from build123d import *

# Parameters (mm, degrees)
F0_R     = 10
F1_DEPTH = 25
F2_DEPTH = 50
F3_SIZE  = 2


with BuildPart() as f1:
    # F0 (on Front) → F1 (new body)
    with BuildSketch(Plane.XZ):
        with BuildLine():
            ThreePointArc((2.083333, -24.913043), (18.399502, -16.92508), (25, 0))
            ThreePointArc((25, 0), (18.399502, 16.92508), (2.083333, 24.913043))
            ThreePointArc((2.083333, 24.913043), (-25, 0), (2.083333, -24.913043))
        make_face()
        Circle(F0_R, mode=Mode.SUBTRACT)
        with BuildLine():
            ThreePointArc((2.083333, 24.913043), (18.399502, 16.92508), (25, 0))
            ThreePointArc((25, 0), (18.399502, -16.92508), (2.083333, -24.913043))
            Line((2.083333, -24.913043), (91.458333, -17.43913))
            ThreePointArc((91.458333, -17.43913), (72.5, 0), (91.458333, 17.43913))
            Line((91.458333, 17.43913), (2.083333, 24.913043))
        make_face()
        with BuildLine():
            ThreePointArc((107.5, 0), (102.879651, 11.847556), (91.458333, 17.43913))
            ThreePointArc((91.458333, 17.43913), (72.5, 0), (91.458333, -17.43913))
            ThreePointArc((91.458333, -17.43913), (102.879651, -11.847556), (107.5, 0))
        make_face()
        with Locations((90, 0)):
            Circle(F0_R, mode=Mode.SUBTRACT)
    extrude(amount=F1_DEPTH)

    # F0 (on Front) → F2 (join)
    with BuildSketch(Plane.XZ):
        with BuildLine():
            ThreePointArc((2.083333, -24.913043), (18.399502, -16.92508), (25, 0))
            ThreePointArc((25, 0), (18.399502, 16.92508), (2.083333, 24.913043))
            ThreePointArc((2.083333, 24.913043), (-25, 0), (2.083333, -24.913043))
        make_face()
        Circle(F0_R, mode=Mode.SUBTRACT)
    extrude(amount=-F2_DEPTH)

    # F3
    f3_edges = [f1.edges().sort_by_distance(p)[0] for p in [
        (-10, 50, 0),
        (-2.083333, 50, 24.913043),
        (80, 0, 0),
    ]]
    chamfer(f3_edges, length=F3_SIZE)


solid = f1.part
Input: part model. Units: mm. Frame: model coordinates. Coordinates: 2 decimals unless noted, no trailing zeros. Loops run counter-clockwise (first coordinate to the right, second up) from the corner with the lowest first, then second, coordinate; pieces in that order, holes last. Notation, with made-up numbers: (-36.5, 74.5) -> (-31.5, 74.5) arc R21 ccw to (-31.5, 80.5) -> close; hole circle Ø11 at (-36, 69.25). An arc over 180 degrees is marked (long way). One line per item, written item: value.
(1) Cut plane A-A (x = 0). Output: boundary loops of the cut face in (y, z).
Answer below:
outline: (-25, -25) -> (48, -25) -> (50, -23) -> (50, -12) -> (48, -10) -> (-25, -10) -> close; (-25, 10) -> (48, 10) -> (50, 12) -> (50, 23) -> (48, 25) -> (-25, 25) -> close
(2) Ray query, line 1 along Z through (x, y) = (0, 22.5); line 2 along Z through (x, y) = (8.5, 1.5); line 3 along Y through (x, z) = (34, 16.5). Return the intervals inside material, ascending.
Answer below:
line 1: z = -25 to -10, 10 to 25
line 2: z = -23.51 to -5.27, 5.27 to 23.51
line 3: y = -25 to 0
(3) Draft query along X for faces 1 (the face through (46.15, -12.32, -21.23)), 2 (the face through (10, 50, -10)), 3 (the face through (80, -13, 0)). Return one class per face: pulls with the +X half, pulls with the -X half, needs draft (parallel to the pull), parting line crosses it, or undercut.
Answer below:
face 1: pulls with the +X half
face 2: needs draft
face 3: undercut
(4) Pin query (flat end, axial travel): pin 1 Ø23 at (x, z) = (0, 0) entering from +Y; pin 2 Ø2 at (y, z) = (21.5, 2.5) entering from +X; pin 3 Ø12 at (x, y) = (20, 9.5) entering from -Z. Return the tip coordinate at first contact, or that it passes through.
Answer below:
pin 1: stops at y = 49.5
pin 2: stops at x = 24.95
pin 3: stops at z = -20.71
(5) Cut plane B-B (y = 8.5). Output: boundary loops of the cut face in (x, z).
Answer below:
outline: (2.08, -24.91) arc R25 ccw to (25, 0) arc R25 ccw to (2.08, 24.91) arc R25 ccw (long way) to start; hole circle Ø20 at (0, 0)
(6) Cut plane C-C (x = 90). Output: boundary loops of the cut face in (y, z), then the cut area to 3 significant figures.
Answer below:
outline: (-25, -17.56) -> (0, -17.56) -> (0, -12) -> (-2, -10) -> (-25, -10) -> close; (-25, 10) -> (-2, 10) -> (0, 12) -> (0, 17.56) -> (-25, 17.56) -> close
area: 374 mm2
(7) Cut plane D-D (x = 35). Output: boundary loops of the cut face in (y, z), then the cut area to 3 significant figures.
Answer below:
outline: (-25, -22.16) -> (0, -22.16) -> (0, 22.16) -> (-25, 22.16) -> close
area: 1,110 mm2
